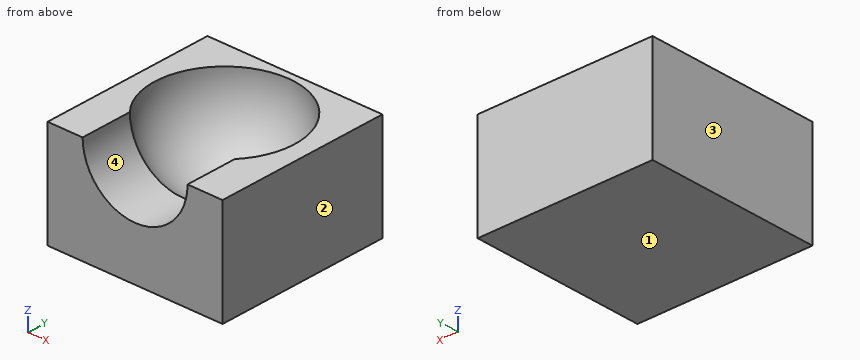
```python
from build123d import *

# Parameters (mm, degrees)
SKETCH1_W           = 25
SKETCH1_H           = 25
BOSS_EXTRUDE1_DEPTH = 15
SKETCH3_R           = 7.5
CUT_EXTRUDE1_DEPTH  = 15


with BuildPart() as part:
    # Sketch1 → Boss-Extrude1 (new body)
    with BuildSketch(Plane.XY):
        with Locations((12.5, 12.5)):
            Rectangle(SKETCH1_W, SKETCH1_H)
    extrude(amount=BOSS_EXTRUDE1_DEPTH)

    # Sketch2 → Cut-Revolve2 (revolve, cut)
    with BuildSketch(Plane.XY.offset(15)):
        with BuildLine():
            Line((12.5, 24), (12.5, 4))
            ThreePointArc((12.5, 4), (22.5, 14), (12.5, 24))
        make_face()
    revolve(axis=Axis((12.5, 24, 15), (0, -1, 0)), mode=Mode.SUBTRACT)

    # Sketch3 → Cut-Extrude1 (cut)
    with BuildSketch(Plane.XZ):
        with Locations((12.5, 15)):
            Circle(SKETCH3_R)
    extrude(amount=-CUT_EXTRUDE1_DEPTH, mode=Mode.SUBTRACT)


solid = part.part
```
The model under review builds one solid part; all positions refer to its coordinate system, in mm. Face numbers are marked on the shaded views. Give positions to 0.01 mm unless a question says otherwise; leave off trailing zeros. Write each loop counter-clockwise with the first axis right and the second up, starting at its lowest first coordinate (ties: lowest second). Pieces come first, ordered by that corner, then holes. Notation, with made-up numbers: M 14.5,49 L 42.5,49 A33 ccw 42.5,81 Z; hole C 14.25,0 d10. An arc over 180 degrees is marked long. Write each question's results on one line, items separated by ' | '. Start each with the question number.
1. Mouldability with a two-part tool opening along X and no side actions: class the marked faces 1, 2, 3 and 4 as released by +X, released by -X, zero draft, split by the parting line, or undercut.
2. Insertion check: pin 1 Ø8 at (x, y) = (14.5, 4.5) entering from +Z. The pin has a flat end and moves straight along its axis. Give the tip position at first contact, or say it passes through.
3. We need section A-A (z = 11.5). Write out the cut boundary in (x, y) (1 decimal), and give its area (3 significant figures).
4. We need section C-C (x = 12.5). Write out the cut boundary in (y, z).
5. For probe 1 along Y at (x, z) = (4.5, 14); probe 2 along X at (y, z) = (4.75, 12.5); probe 3 along X at (y, z) = (15.75, 14), list the stretches that pass through material, from the lowest coordinate up. Write a range as [from, to].
6. We need section B-B (y = 20). Write out the cut boundary in (x, z).
7. We need section D-D (z = 5.75). Write out the cut boundary in (x, y).
Results found:
1) face 1: zero draft | face 2: released by +X | face 3: released by -X | face 4: undercut
2) pin 1: stops at z = 10.5
3) outline: M 0,0 L 5.9,0 L 5.9,7.4 A9.4 cw long 19.1,7.4 L 19.1,0 L 25,0 L 25,25 L 0,25 Z | area: 277 mm^2
4) outline: M 0,0 L 25,0 L 25,15 L 24,15 A10 cw 7.39,7.5 L 0,7.5 Z
5) probe 1: y = [0, 8.08], [19.92, 25] | probe 2: x = [0, 5.43], [19.57, 25] | probe 3: x = [0, 2.71], [22.29, 25]
6) outline: M 0,0 L 25,0 L 25,15 L 20.5,15 A8 cw 4.5,15 L 0,15 Z
7) outline: M 0,0 L 25,0 L 25,25 L 0,25 Z; hole C 12.5,14 d7.6
